Design review of the part built by this model. Coordinates are the model's own, in mm. A direction names the side the tool comes from. Give positions to 0.01 mm unless a question says otherwise; leave off trailing zeros. Order: outer loops, then holes, each group sorted by start corner. A loop starts at its lowest first (then second) coordinate and runs counter-clockwise, first axis right, second up. Notation, with made-up numbers: (-7.75, -14) - (32.25, -14) arc R16 cw to (32.25, -4) - close; hole circle Ø4 at (4, 28.25). An arc over 180 degrees is marked (long way). Write each question's results on one line, items separated by ' | '. Start each with the question number.
```python
from build123d import *

# Parameters (mm, degrees)
SKETCH006_W     = 97
SKETCH006_H     = 66
SKETCH006_R     = 1.5
SKETCH006_W_2   = 13
SKETCH006_H_2   = 27
PAD004_DEPTH    = 2
SKETCH007_W     = 97
SKETCH007_H     = 66
SKETCH007_W_2   = 93
SKETCH007_H_2   = 62
PAD005_DEPTH    = 18
SKETCH008_R     = 2.7
SKETCH008_R_2   = 1.5
PAD006_DEPTH    = 4
SKETCH012_W     = 13
SKETCH012_H     = 8
POCKET001_DEPTH = 2
SKETCH026_W     = 20
SKETCH026_H     = 15
POCKET007_DEPTH = 2


with BuildPart() as part:
    # Sketch006 → Pad004 (new body)
    with BuildSketch(Plane.XY):
        with Locations((48.5, 33)):
            Rectangle(SKETCH006_W, SKETCH006_H)
        with Locations((87.5, 57.5)):
            Circle(SKETCH006_R, mode=Mode.SUBTRACT)
        with Locations((87.5, 8.5)):
            Circle(SKETCH006_R, mode=Mode.SUBTRACT)
        with Locations((29.5, 57.5)):
            Circle(SKETCH006_R, mode=Mode.SUBTRACT)
        with Locations((29.5, 8.5)):
            Circle(SKETCH006_R, mode=Mode.SUBTRACT)
        with Locations((48.5, 33)):
            Rectangle(SKETCH006_W_2, SKETCH006_H_2, mode=Mode.SUBTRACT)
    extrude(amount=PAD004_DEPTH)

    # Sketch007 → Pad005 (join)
    with BuildSketch(Plane.XY):
        with Locations((48.5, 33)):
            Rectangle(SKETCH007_W, SKETCH007_H)
        with Locations((48.5, 33)):
            Rectangle(SKETCH007_W_2, SKETCH007_H_2, mode=Mode.SUBTRACT)
    extrude(amount=PAD005_DEPTH)

    # Sketch008 → Pad006 (join)
    with BuildSketch(Plane.XY):
        with Locations((29.5, 57.5)):
            Circle(SKETCH008_R)
        with Locations((29.5, 57.5)):
            Circle(SKETCH008_R_2, mode=Mode.SUBTRACT)
        with Locations((87.5, 57.5)):
            Circle(SKETCH008_R)
        with Locations((87.5, 57.5)):
            Circle(SKETCH008_R_2, mode=Mode.SUBTRACT)
        with Locations((87.5, 8.5)):
            Circle(SKETCH008_R)
        with Locations((87.5, 8.5)):
            Circle(SKETCH008_R_2, mode=Mode.SUBTRACT)
        with Locations((29.5, 8.5)):
            Circle(SKETCH008_R)
        with Locations((29.5, 8.5)):
            Circle(SKETCH008_R_2, mode=Mode.SUBTRACT)
    extrude(amount=PAD006_DEPTH)

    # Sketch012 → Pocket001 (cut)
    with BuildSketch(Plane(origin=(74, 66, 4), x_dir=(1, 0, 0), z_dir=(0, -1, 0))):
        with Locations((6.5, 4)):
            Rectangle(SKETCH012_W, SKETCH012_H)
    extrude(amount=POCKET001_DEPTH, mode=Mode.SUBTRACT)

    # Sketch026 → Pocket007 (cut)
    with BuildSketch(Plane.YZ):
        with Locations((32, 10.5)):
            Rectangle(SKETCH026_W, SKETCH026_H)
    extrude(amount=POCKET007_DEPTH, mode=Mode.SUBTRACT)


solid = part.part
```
Q1. Add section A-A (x = 29.5). Give the boundary of the cut face in (y, z).
Q2. Machinability: for faces 4 (the flat face through (48, 19.5, 1)), 5 (the flat face through (89, 56, 4)), 6 (the flat face through (80, 65, 4)), which of the approach directions +Z, -Z, +X, -X, +Y, -Y give a long, thin tool a straight path to every point of the face, cutting with its end or side? Answer none if there is none.
Q3. Insertion check: pin 1 Ø6 at (x, y) = (29, 58.5) entering from +Z; pin 2 Ø2 at (x, z) = (45.5, 1) entering from -Y; pin 3 Ø6 at (x, y) = (28, 15.5) entering from +Z; pin 4 Ø2.5 at (x, y) = (87.5, 57.5) entering from +Z. Each pin has a flat end and moves straight along its axis. Give the tip position at first contact, or say it passes through.
Q4. Add section D-D (x = 78). Give the boundary of the cut face in (y, z), plus the area to 3 significant figures.
Q5. Draft analysis for pull direction Y (two halves, no side actions). For faces 1 (the flat face through (80, 65, 12)), 2 (the flat face through (48, 66, 9)), 3 (the flat face through (1, 42, 10)), state which applies: pulls with the +Y half, pulls with the -Y half, needs draft (parallel to the pull), parting line crosses it, or undercut.
Q6. Add section B-B (y = 34.5). Give the boundary of the cut face in (x, z).
Q7. For line 1 (Y direction, x = 87.5, z = 3); line 2 (Y direction, x = 87.5, z = 1.8); line 3 (Y direction, x = 45, z = 5), list the stretches that pass through material, from the lowest coordinate up. Write a range as [from, to].
Q8. Add section C-C (y = 8.5). Give the boundary of the cut face in (x, z), plus the area to 3 significant figures.
Verdict:
1) outline: (0, 0) - (7, 0) - (7, 4) - (5.8, 4) - (5.8, 2) - (2, 2) - (2, 18) - (0, 18) - close; (10, 0) - (56, 0) - (56, 4) - (54.8, 4) - (54.8, 2) - (11.2, 2) - (11.2, 4) - (10, 4) - close; (59, 0) - (66, 0) - (66, 18) - (64, 18) - (64, 2) - (60.2, 2) - (60.2, 4) - (59, 4) - close
2) face 4: +Z, -Z | face 5: +Z | face 6: +Y
3) pin 1: stops at z = 4 | pin 2: stops at y = 0 | pin 3: stops at z = 2 | pin 4: passes through
4) outline: (0, 0) - (66, 0) - (66, 4) - (64, 4) - (64, 2) - (2, 2) - (2, 18) - (0, 18) - close; (64, 12) - (66, 12) - (66, 18) - (64, 18) - close | area: 180 mm2
5) face 1: needs draft | face 2: pulls with the +Y half | face 3: undercut
6) outline: (0, 0) - (42, 0) - (42, 2) - (2, 2) - (2, 3) - (0, 3) - close; (55, 0) - (97, 0) - (97, 18) - (95, 18) - (95, 2) - (55, 2) - close
7) line 1: y = [0, 2], [5.8, 7], [10, 11.2], [54.8, 56], [59, 60.2], [64, 66] | line 2: y = [0, 7], [10, 56], [59, 66] | line 3: y = [0, 2], [64, 66]
8) outline: (0, 0) - (28, 0) - (28, 4) - (26.8, 4) - (26.8, 2) - (2, 2) - (2, 18) - (0, 18) - close; (31, 0) - (86, 0) - (86, 4) - (84.8, 4) - (84.8, 2) - (32.2, 2) - (32.2, 4) - (31, 4) - close; (89, 0) - (97, 0) - (97, 18) - (95, 18) - (95, 2) - (90.2, 2) - (90.2, 4) - (89, 4) - close | area: 256 mm2
